For this review, take the finished solid that the model builds, in its own axes (mm). A direction names the side the tool comes from. Coordinates: 2 decimals unless noted, no trailing zeros. Write each loop counter-clockwise with the first axis right and the second up, starting at its lowest first coordinate (ties: lowest second). Pieces come first, ordered by that corner, then holes. Notation, with made-up numbers: M -23,-27 L 32,-27 A28 cw 32,0 Z; hole C -3.5,76 d9. An arc over 180 degrees is marked long. Return JSON: item names as keys, results as strings.
```python
from build123d import *

# Parameters (mm, degrees)
F0_R     = 7.62
F0_W     = 5.08
F0_H     = 0.508
F1_DEPTH = 6.35
F2_T     = -1.27
F3_R     = 2.53999
F4_R     = 1.26999


# Not quite as in the source:
# - a fillet or chamfer is up to 0.001 mm smaller than in the source, because OpenCascade refuses the exact size


with BuildPart() as f1:
    # F0 (on Right) → F1 (new body, symmetric)
    with BuildSketch(Plane.YZ):
        with BuildLine():
            Line((-15.24, 15.24), (-25.4, 15.24))
            Line((-25.4, 15.24), (-25.4, 10.16))
            Line((-25.4, 10.16), (-15.24, 10.16))
            Line((-15.24, 10.16), (-15.24, 0))
            ThreePointArc((-15.24, 0), (10.7763073453, -10.7763073453), (0, 15.24))
            Line((0, 15.24), (-10.16, 15.24))
            Line((-10.16, 15.24), (-15.24, 15.24))
        make_face()
        Circle(F0_R, mode=Mode.SUBTRACT)
        with Locations((-12.7, 15.494)):
            Rectangle(F0_W, F0_H)
    extrude(amount=F1_DEPTH, both=True)

    # F2
    f2_openings = [f1.faces().sort_by_distance(p)[0] for p in [
        (0, -25.4, 12.7),
        (0, -12.7, 15.748),
    ]]
    offset(amount=F2_T, openings=f2_openings, kind=Kind.INTERSECTION)

    # F3 (radius 2.54 in the source; OpenCascade refuses exactly that, so slightly less here)
    f3_edges = [f1.edges().sort_by_distance(p)[0] for p in [
        (-6.35, -20.32, 15.24),
        (-6.35, -20.32, 10.16),
        (6.35, -20.32, 15.24),
        (6.35, -20.32, 10.16),
    ]]
    fillet(f3_edges, radius=F3_R)

    # F4 (radius 1.27 in the source; OpenCascade refuses exactly that, so slightly less here)
    f4_edges = [f1.edges().sort_by_distance(p)[0] for p in [
        (-5.08, -19.685, 11.43),
        (-5.08, -19.685, 13.97),
        (5.08, -19.685, 13.97),
        (5.08, -19.685, 11.43),
    ]]
    fillet(f4_edges, radius=F4_R)


solid = f1.part
```
1. For faces 1 (the face through (-5.6, -20.4, 14.5)), 2 (the face through (0, -20, 13.97)), 3 (the face through (0, -13.97, 15)), 4 (the face through (0.071, 9.547, -10.199)), list the 3-axis set-ups (+Z, -Z, +X, -X, +Y, -Y) from which the entire face can be reached by the end or side of a thin tool; tool diameter is ignored.
Checks:
{"face 1": "+Z, -X, -Y", "face 2": "-Y", "face 3": "+Z", "face 4": "none"}
2. Wall thickness on L1, parallel to X at y = -10, z = 5; L2, parallel to Y at x = 3.25, z = -4; L3, parallel to Y at x = -1.25, z = 6.5: over which ranges is each line inside the solid? List them lowest first. Write a range as from..to.
Checks:
{"L1": "-6.35..-5.08, 5.08..6.35", "L2": "-14.71..-13.39, -7.94..-6.49, 6.49..7.94, 13.39..14.71", "L3": "-15.24..-13.97, -6.06..-3.98, 3.98..6.06, 12.37..13.78"}
3. We need section D-D (y = 11). State the section outline as (x, z) points, plus the area to 3 significant figures.
Checks:
{"outline": "M -6.35,-10.55 L 6.35,-10.55 L 6.35,10.55 L -6.35,10.55 Z; hole M -5.08,-8.61 L 5.08,-8.61 L 5.08,8.61 L -5.08,8.61 Z", "area": "92.9 mm2"}
4. We need section B-B (z = 2). State the section outline as (x, y) points.
Checks:
{"outline": "M -6.35,-15.24 L 6.35,-15.24 L 6.35,-7.35 L -6.35,-7.35 Z; M -6.35,7.35 L 6.35,7.35 L 6.35,15.11 L -6.35,15.11 Z; hole M -5.08,-13.97 L 5.08,-13.97 L 5.08,-8.66 L -5.08,-8.66 Z; hole M -5.08,8.66 L 5.08,8.66 L 5.08,13.83 L -5.08,13.83 Z"}
5. Draft analysis for pull direction Z (two halves, no side actions). For faces 5 (the face through (-5.08, -3, 9)), 6 (the face through (0, -11.43, 15)), 7 (the face through (5.6, -20.4, 14.5)), state which applies: +Z half, -Z half, draft (parallel to the pull), parting line (faces both ways), or undercut.
Checks:
{"face 5": "undercut", "face 6": "draft", "face 7": "+Z half"}
6. Clearance check with flat-ended pins moving along their axes: pin 1 Ø2.5 at (x, z) = (-2, 15) entering from +Y; pin 2 Ø2 at (x, z) = (2, 0) entering from -Y; pin 3 Ø1.5 at (x, y) = (-1.5, -5) entering from -Z. State where each tip first meets the part, or that it passes through.
Checks:
{"pin 1": "y = 6.57", "pin 2": "y = -15.24", "pin 3": "z = -14.64"}
7. We need section A-A (x = 1.5). State the section outline as (y, z) points.
Checks:
{"outline": "M -25.4,10.16 L -15.24,10.16 L -15.24,0 A15.24 ccw long 0,15.24 L -10.16,15.24 L -10.16,15.75 L -11.43,15.75 L -11.43,13.97 L 0,13.97 A13.97 cw long -13.97,0 L -13.97,11.43 L -25.4,11.43 Z; M -25.4,13.97 L -13.97,13.97 L -13.97,15.75 L -15.24,15.75 L -15.24,15.24 L -25.4,15.24 Z; C 0,0 d17.78; hole C 0,0 d15.24"}
8. We need section C-C (y = 1). State the section outline as (x, z) points.
Checks:
{"outline": "M -6.35,-15.21 L 6.35,-15.21 L 6.35,-7.55 L -6.35,-7.55 Z; M -6.35,7.55 L 6.35,7.55 L 6.35,15.21 L -6.35,15.21 Z; hole M -5.08,-13.93 L 5.08,-13.93 L 5.08,-8.83 L -5.08,-8.83 Z; hole M -5.08,8.83 L 5.08,8.83 L 5.08,13.93 L -5.08,13.93 Z"}
